Verification items for the finished model (mm, model axes). Face numbers are marked on the shaded views. A direction names the side the tool comes from. Coordinates: 2 decimals unless noted, no trailing zeros. Write each loop counter-clockwise with the first axis right and the second up, starting at its lowest first coordinate (ties: lowest second). Pieces come first, ordered by that corner, then holes. Notation, with made-up numbers: (43, -9.5) -> (89, -9.5) arc R25 cw to (89, 18.5) -> close; hole circle Ø9 at (38.25, 37). An arc over 180 degrees is marked (long way). Answer in a Markdown table with one row per item.
```python
from build123d import *

# Parameters (mm, degrees)
SKETCH4_W           = 40
SKETCH4_H           = 24
BOSS_EXTRUDE2_DEPTH = 3.5
FILLET2_R           = 1
SKETCH5_W           = 4.999999906
SKETCH5_H           = 14
BOSS_EXTRUDE3_DEPTH = 2
FILLET3_R           = 1
CHAMFER1_SIZE       = 2.8
SKETCH6_R           = 1.15
CUT_EXTRUDE1_DEPTH  = 5
SKETCH8_R           = 0.6
CUT_EXTRUDE2_DEPTH  = 1.75
SKETCH9_R           = 3.5
CUT_EXTRUDE3_DEPTH  = 1.5
SKETCH10_R          = 3
CUT_EXTRUDE4_DEPTH  = 1
CUT_EXTRUDE5_DEPTH  = 0.8
SKETCH12_R          = 2.5
CUT_EXTRUDE6_DEPTH  = 1
CUT_EXTRUDE7_DEPTH  = 0.8
CUT_EXTRUDE8_DEPTH  = 0.8
SKETCH16_R          = 2.25
CUT_EXTRUDE9_DEPTH  = 1.5
CUT_EXTRUDE10_DEPTH = 0.5
SKETCH18_R          = 0.5
CUT_EXTRUDE11_DEPTH = 47.70385414
LPATTERN3_COUNT     = 4
LPATTERN3_PITCH     = 6


with BuildPart() as part:
    # Sketch4 → Boss-Extrude2 (new body)
    with BuildSketch(Plane(origin=(0, 0, 0), x_dir=(1, 0, 0), z_dir=(0, 1, 0))):
        with Locations((20, 0)):
            Rectangle(SKETCH4_W, SKETCH4_H)
    extrude(amount=BOSS_EXTRUDE2_DEPTH)

    # Fillet2
    fillet2_edges = [part.edges().sort_by_distance(p)[0] for p in [
        (40, 1.75, -12),
        (40, 1.75, 12),
        (0, 1.75, 12),
    ]]
    fillet(fillet2_edges, radius=FILLET2_R)

    # Sketch5 → Boss-Extrude3 (add)
    with BuildSketch(Plane(origin=(0, 3.5, 0), x_dir=(1, 0, 0), z_dir=(0, 1, 0))):
        with Locations((42.499999953, 0)):
            Rectangle(SKETCH5_W, SKETCH5_H)
    extrude(amount=-BOSS_EXTRUDE3_DEPTH)

    # Fillet3
    fillet3_edges = [part.edges().sort_by_distance(p)[0] for p in [
        (44.999999906, 2.5, -7),
        (44.999999906, 2.5, 7),
    ]]
    fillet(fillet3_edges, radius=FILLET3_R)

    # Chamfer1
    chamfer1_edges = [part.edges().sort_by_distance(p)[0] for p in [
        (0, 1.75, -12),
    ]]
    chamfer(chamfer1_edges, length=CHAMFER1_SIZE)

    # Sketch6 → Cut-Extrude1 (cut)
    with BuildSketch(Plane.ZY):
        with Locations((0, 1.75)):
            Circle(SKETCH6_R)
    extrude(amount=-CUT_EXTRUDE1_DEPTH, mode=Mode.SUBTRACT)

    # Sketch8 → Cut-Extrude2 (cut)
    with BuildSketch(Plane.XZ):
        with Locations(Location((5, 0, 0), (0, 0, 270))):
            Circle(SKETCH8_R)
    extrude(amount=-CUT_EXTRUDE2_DEPTH, mode=Mode.SUBTRACT)

    # Sketch9 → Cut-Extrude3 (cut)
    with BuildSketch(Plane.XZ):
        with Locations(Location((7, 0, 0), (0, 0, 270))):
            Circle(SKETCH9_R)
    extrude(amount=-CUT_EXTRUDE3_DEPTH, mode=Mode.SUBTRACT)

    # Sketch10 → Cut-Extrude4 (cut)
    with BuildSketch(Plane.XZ):
        with Locations(Location((7, -7, 0), (0, 0, 270))):
            Circle(SKETCH10_R)
    extrude(amount=-CUT_EXTRUDE4_DEPTH, mode=Mode.SUBTRACT)

    # Sketch11 → Cut-Extrude5 (cut)
    with BuildSketch(Plane(origin=(0, 0, 0), x_dir=(-1, 0, 0), z_dir=(0, -1, 0))):
        with BuildLine():
            Line((-6.5, 7), (-6.5, 3.5))
            ThreePointArc((-6.5, 3.5), (-7, 3), (-7.5, 3.5))
            Line((-7.5, 3.5), (-7.5, 7))
            ThreePointArc((-7.5, 7), (-7, 7.5), (-6.5, 7))
        make_face()
        with BuildLine():
            Line((-20, 0.5), (-7, 0.5))
            ThreePointArc((-7, 0.5), (-6.5, 0), (-7, -0.5))
            Line((-7, -0.5), (-20, -0.5))
            ThreePointArc((-20, -0.5), (-20.5, 0), (-20, 0.5))
        make_face()
    extrude(amount=-CUT_EXTRUDE5_DEPTH, mode=Mode.SUBTRACT)

    # Sketch12 → Cut-Extrude6 (cut)
    with BuildSketch(Plane.XZ):
        with Locations(Location((14, 0, 0), (0, 0, 270))):
            Circle(SKETCH12_R)
    extrude(amount=-CUT_EXTRUDE6_DEPTH, mode=Mode.SUBTRACT)

    # Sketch14 → Cut-Extrude7 (cut)
    with BuildSketch(Plane.XZ):
        with BuildLine():
            Line((19.5, -9), (19.5, 9))
            ThreePointArc((19.5, 9), (20, 9.5), (20.5, 9))
            Line((20.5, 9), (20.5, -9))
            ThreePointArc((20.5, -9), (20, -9.5), (19.5, -9))
        make_face()
    extrude(amount=-CUT_EXTRUDE7_DEPTH, mode=Mode.SUBTRACT)

    # Sketch15 → Cut-Extrude8 (cut)
    with BuildSketch(Plane.XZ):
        with BuildLine():
            Line((20, -8.5), (24, -8.5))
            ThreePointArc((24, -8.5), (24.5, -9), (24, -9.5))
            Line((24, -9.5), (20, -9.5))
            ThreePointArc((20, -9.5), (19.5, -9), (20, -8.5))
        make_face()
    cut_extrude8 = extrude(amount=-CUT_EXTRUDE8_DEPTH, mode=Mode.SUBTRACT)

    # Sketch16 → Cut-Extrude9 (cut)
    with BuildSketch(Plane.XZ):
        with Locations(Location((24, -9, 0), (0, 0, 270))):
            Circle(SKETCH16_R)
    cut_extrude9 = extrude(amount=-CUT_EXTRUDE9_DEPTH, mode=Mode.SUBTRACT)

    # Sketch17 → Cut-Extrude10 (cut)
    with BuildSketch(Plane.XZ):
        with BuildLine():
            Line((31, -9.3), (24, -9.3))
            ThreePointArc((24, -9.3), (23.7, -9), (24, -8.7))
            Line((24, -8.7), (31, -8.7))
            ThreePointArc((31, -8.7), (31.3, -9), (31, -9.3))
        make_face()
    cut_extrude10 = extrude(amount=-CUT_EXTRUDE10_DEPTH, mode=Mode.SUBTRACT)

    # Sketch18 → Cut-Extrude11 (cut, through all)
    with BuildSketch(Plane(origin=(0, 0, 0), x_dir=(-1, 0, 0), z_dir=(0, -1, 0))):
        with Locations(Location((-31, 9, 0), (0, 0, 90))):
            Circle(SKETCH18_R)
    cut_extrude11 = extrude(amount=-CUT_EXTRUDE11_DEPTH, mode=Mode.SUBTRACT)

    # LPattern3: Cut-Extrude8, Cut-Extrude9, Cut-Extrude10, Cut-Extrude11 ×4
    with Locations(*[(0, 0, i * LPATTERN3_PITCH) for i in range(1, LPATTERN3_COUNT)]):
        add(cut_extrude8, mode=Mode.SUBTRACT)
        add(cut_extrude9, mode=Mode.SUBTRACT)
        add(cut_extrude10, mode=Mode.SUBTRACT)
        add(cut_extrude11, mode=Mode.SUBTRACT)


solid = part.part
```
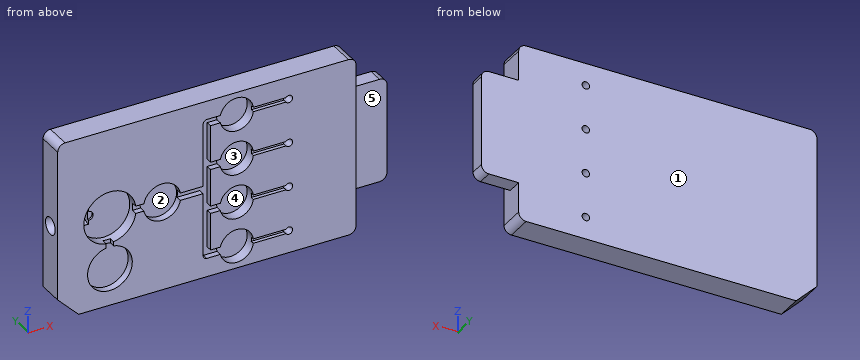
1. Sectioned sample at A-A, the plane z = 0. Record the cut outline in (x, y).
Findings below:
| item | result |
|---|---|
| outline | (0, 0) -> (3.5, 0) -> (3.5, 0.6) -> (0, 0.6) -> close; (0, 2.9) -> (5, 2.9) -> (5, 1.75) -> (5.6, 1.75) -> (5.6, 1.5) -> (10.5, 1.5) -> (10.5, 0.8) -> (11.5, 0.8) -> (11.5, 1) -> (16.5, 1) -> (16.5, 0.8) -> (20.5, 0.8) -> (20.5, 0) -> (40, 0) -> (40, 1.5) -> (45, 1.5) -> (45, 3.5) -> (0, 3.5) -> close |
2. Sectioned sample at D-D, the plane x = 14. Record the cut outline in (y, z), and give its area (3 significant figures).
Findings below:
| item | result |
|---|---|
| outline | (0, -12) -> (3.5, -12) -> (3.5, 12) -> (0, 12) -> (0, 2.5) -> (1, 2.5) -> (1, -2.5) -> (0, -2.5) -> close |
| area | 79.0 mm² |
3. Material ranges on probe 1 along Z at (x, y) = (24, 0.7); probe 2 along Y at (x, z) = (1.1, 0); probe 3 along Z at (x, y) = (31, 0.75), recorded low to high. Write a range as from..to.
Findings below:
| item | result |
|---|---|
| probe 1 | z = -12..-11.25, -6.75..-5.25, -0.75..0.75, 5.25..6.75, 11.25..12 |
| probe 2 | y = 0..0.6, 2.9..3.5 |
| probe 3 | z = -12..-9.5, -8.5..-3.5, -2.5..2.5, 3.5..8.5, 9.5..12 |
4. Sectioned sample at B-B, the plane x = 24. Record the cut outline in (y, z), and give its area (3 significant figures).
Findings below:
| item | result |
|---|---|
| outline | (0, -12) -> (3.5, -12) -> (3.5, 12) -> (0, 12) -> (0, 11.25) -> (1.5, 11.25) -> (1.5, 6.75) -> (0, 6.75) -> (0, 5.25) -> (1.5, 5.25) -> (1.5, 0.75) -> (0, 0.75) -> (0, -0.75) -> (1.5, -0.75) -> (1.5, -5.25) -> (0, -5.25) -> (0, -6.75) -> (1.5, -6.75) -> (1.5, -11.25) -> (0, -11.25) -> close |
| area | 57.0 mm² |
5. Sectioned sample at C-C, the plane z = 8. Record the cut outline in (x, y), and give its area (3 significant figures).
Findings below:
| item | result |
|---|---|
| outline | (0, 0) -> (19.5, 0) -> (19.5, 0.8) -> (20.5, 0.8) -> (20.5, 0) -> (21.98, 0) -> (21.98, 1.5) -> (26.02, 1.5) -> (26.02, 0) -> (40, 0) -> (40, 3.5) -> (0, 3.5) -> close |
| area | 133 mm² |
6. Go/stop test with flat-tipped pins: pin 1 (1.3 mm diameter, centred on x = 25, z = -3, fed in from -Y); pin 2 (1.8 mm diameter, centred on y = 1.75, z = 0, fed in from -X). Record where each tip stops, or that it passes through.
Findings below:
| item | result |
|---|---|
| pin 1 | stops at y = 1.5 |
| pin 2 | stops at x = 5 |
7. Release check for a two-part mould opening along X. For the marked faces 3, 4 and 5 record: released by +X, released by -X, zero draft, split by the parting line, or undercut.
Findings below:
| item | result |
|---|---|
| face 3 | undercut |
| face 4 | undercut |
| face 5 | zero draft |
8. Access from +Z, -Z, +X, -X, +Y, -Y to the whole of each face (thin tool, end or side, straight path). Record for the marked faces 1 and 2.
Findings below:
| item | result |
|---|---|
| face 1 | +Z, -Z, +X, -X, +Y |
| face 2 | -Y |
